Source: CAD feature listing. Evaluate the final solid. Frame: model axes, mm. A direction names the side the tool comes from. Give positions to 0.01 mm unless a question says otherwise; leave off trailing zeros. Loops run counter-clockwise (first coordinate to the right, second up) from the corner with the lowest first, then second, coordinate; pieces in that order, holes last.
Autodesk Inventor part; units mm, degrees
ref_plane "YZ Plane" through (0, 0, 0) normal (1, 0, 0) x (0, 1, 0)
ref_plane "XZ Plane" through (0, 0, 0) normal (0, 1, 0) x (-1, 0, 0)
ref_plane "XY Plane" through (0, 0, 0) normal (0, 0, 1) x (1, 0, 0)
sketch "Boceto1" plane through (0, 0, 0) normal (0, 0, 1) x (1, 0, 0)
  point P0 (0, 0)
sketch "Boceto2" plane through (0, 0, 0) normal (0, 0, 1) x (1, 0, 0)
  line L0 (12, 0) -> (28, 0)
  line L1 (40, 12) -> (40, 228)
  line L2 (28, 240) -> (12, 240)
  line L3 (0, 228) -> (0, 12)
  arc A0 (12, 240) -> (0, 228) centre (12, 228) ccw
  arc A1 (40, 228) -> (28, 240) centre (28, 228) ccw
  circle A2 centre (20, 20) radius 5
  line L4 (20, 40) -> (20, 40)
  line L5 (30, 50) -> (30, 220)
  line L6 (20, 230) -> (20, 230)
  line L7 (10, 220) -> (10, 50)
  line L8 (10, 40) -> (30, 230) construction
  line L9 (30, 40) -> (10, 230) construction
  arc A3 (0, 12) -> (12, 0) centre (12, 12) ccw
  arc A4 (28, 0) -> (40, 12) centre (28, 12) ccw
  arc A5 (10, 50) -> (20, 40) centre (20, 50) ccw
  arc A6 (20, 40) -> (30, 50) centre (20, 50) ccw
  arc A7 (20, 230) -> (10, 220) centre (20, 220) ccw
  arc A8 (30, 220) -> (20, 230) centre (20, 220) ccw
  point P0 (0, 0)
  point P1 (40, 240)
  point P2 (40, 0)
  point P3 (0, 240)
  point P4 (20, 0)
  point P5 (20, 135)
  point P6 (20, 40)
  point P7 (20, 230)
  point P8 (20, 240)
  dimension "d0" = 40
  dimension "d1" = 240
  dimension "d2" = 12
  dimension "d3" = 12
  dimension "d4" = 10
  dimension "d5" = 20
  dimension "d6" = 20
  dimension "d7" = 190
  dimension "d9" = 12
  dimension "d10" = 10
  dimension "d14" = 200
extrude "Extrusión1" add sketch "Boceto2" along normal blind 6
properties part number "Eslabon 2"
(1) Section B-B, the plane x = 20. Return the cut outline in (y, z).
A:
outline: (0, 0) - (15, 0) - (15, 6) - (0, 6) - close; (25, 0) - (40, 0) - (40, 6) - (25, 6) - close; (230, 0) - (240, 0) - (240, 6) - (230, 6) - close
(2) Section D-D, the plane y = 20. Return the cut outline in (x, z).
A:
outline: (0, 0) - (15, 0) - (15, 6) - (0, 6) - close; (25, 0) - (40, 0) - (40, 6) - (25, 6) - close
(3) First-contact query: pin 1 (3 mm diameter, centred on y = 126, z = 2.5, fed in from -X). Flat tip, straight axial feed; report the tip coordinate or a pass-through.
A:
pin 1: stops at x = 0
(4) Section C-C, the plane z = 2.6. Return the cut outline in (x, y), then the cut area to 3 significant figures.
A:
outline: (0, 12) arc R12 ccw to (12, 0) - (28, 0) arc R12 ccw to (40, 12) - (40, 228) arc R12 ccw to (28, 240) - (12, 240) arc R12 ccw to (0, 228) - close; hole (10, 50) arc R10 ccw to (30, 50) - (30, 220) arc R10 ccw to (10, 220) - close; hole circle Ø10 at (20, 20)
area: 5,680 mm2
(5) Mould query, pull axis X, two halves, no side actions, for faces 1 (the flat face through (20, 240, 3)), 2 (the cylindrical face through (36.39, 236.58, 2.96)), 3 (the cylindrical face through (18.92, 24.88, 2.96)). Classes: pulls with the +X half, pulls with the -X half, needs draft (parallel to the pull), parting line crosses it, or undercut.
A:
face 1: needs draft
face 2: pulls with the +X half
face 3: undercut
(6) Reachability of faces 4 (the cylindrical face through (20, 40, 3)), 5 (the flat face through (0, 122, 3)) from +Z, -Z, +X, -X, +Y, -Y: full face, straight path, thin tool, end or side. Return the list, or none.
A:
face 4: +Z, -Z
face 5: +Z, -Z, -X, +Y, -Y
(7) Ray query, line 1 along Y through (x, z) = (20, 2.25); line 2 along X through (y, z) = (190, 2.7); line 3 along Y through (x, z) = (17, 5.55). Return the intervals inside material, ascending.
A:
line 1: y = 0 to 15, 25 to 40, 230 to 240
line 2: x = 0 to 10, 30 to 40
line 3: y = 0 to 16, 24 to 40.46, 229.54 to 240
(8) Section A-A, the plane y = 161.5. Return the cut outline in (x, z), then the cut area to 3 significant figures.
A:
outline: (0, 0) - (10, 0) - (10, 6) - (0, 6) - close; (30, 0) - (40, 0) - (40, 6) - (30, 6) - close
area: 120 mm2
